Geometry check sheet. Reference: the model listing, model coordinates, mm. Face numbers are marked on the shaded views. A direction names the side the tool comes from. Round coordinates to 2 decimals unless told otherwise and drop trailing zeros. Write each loop counter-clockwise with the first axis right and the second up, starting at its lowest first coordinate (ties: lowest second). Pieces come first, ordered by that corner, then holes. Notation, with made-up numbers: M 74.25,-40 L 121.25,-40 A36 ccw 121.25,-3 Z; hole C 83.25,33 d11. An arc over 180 degrees is marked long. Use a Markdown table: item, result.
```python
from build123d import *

# Parameters (mm, degrees)
F0_W     = 25.4
F0_H     = 5.9481007091
F1_DEPTH = 12.7
F2_DEPTH = 25.4


with BuildPart() as f1:
    # F0 (on Front) → F1 (new body)
    with BuildSketch(Plane.XZ):
        with Locations((-12.7, 2.9740503545)):
            Rectangle(F0_W, F0_H)
        with BuildLine():
            Line((-25.4, 11.7354422192), (-25.4, 5.9481007091))
            Line((-25.4, 5.9481007091), (0, 5.9481007091))
            Line((0, 5.9481007091), (0, 11.7354422192))
            ThreePointArc((0, 11.7354422192), (-12.7, 24.4354422192), (-25.4, 11.7354422192))
        make_face()
    extrude(amount=-F1_DEPTH)

    # F0 (on Front) → F2 (join)
    with BuildSketch(Plane.XZ):
        with Locations((-12.7, 2.9740503545)):
            Rectangle(F0_W, F0_H)
    extrude(amount=F2_DEPTH)


solid = f1.part
```
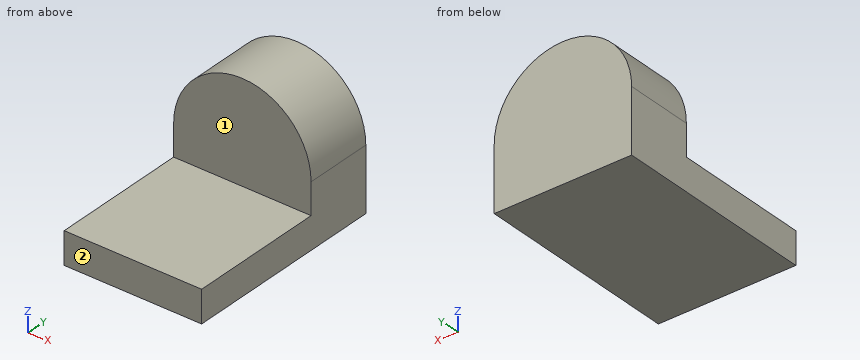
Item 1: Access from +Z, -Z, +X, -X, +Y, -Y to the whole of each face (thin tool, end or side, straight path). Record for the marked faces 1 and 2.
Outcome:
| item | result |
|---|---|
| face 1 | +Z, +X, -X, -Y |
| face 2 | +Z, -Z, +X, -X, -Y |
Item 2: Cross-section at C-C, the plane y = -7. Record the cut outline in (x, z).
Outcome:
| item | result |
|---|---|
| outline | M -25.4,0 L 0,0 L 0,5.95 L -25.4,5.95 Z |
Item 3: Material ranges on line 1 along Z through (x, y) = (-7.25, -7.5); line 2 along Y through (x, z) = (-1.25, 10); line 3 along Z through (x, y) = (-17.5, 3.5), recorded low to high. Write a range as from..to.
Outcome:
| item | result |
|---|---|
| line 1 | z = 0..5.95 |
| line 2 | y = 0..12.7 |
| line 3 | z = 0..23.49 |
Item 4: Cross-section at A-A, the plane x = -12.7. Record the cut outline in (y, z), and give its area (3 significant figures).
Outcome:
| item | result |
|---|---|
| outline | M -25.4,0 L 12.7,0 L 12.7,24.44 L 0,24.44 L 0,5.95 L -25.4,5.95 Z |
| area | 461 mm2 |
Item 5: Cross-section at D-D, the plane x = -4.5. Record the cut outline in (y, z).
Outcome:
| item | result |
|---|---|
| outline | M -25.4,0 L 12.7,0 L 12.7,21.43 L 0,21.43 L 0,5.95 L -25.4,5.95 Z |
Item 6: Cross-section at B-B, the plane z = 18. Record the cut outline in (x, y).
Outcome:
| item | result |
|---|---|
| outline | M -23.75,0 L -1.65,0 L -1.65,12.7 L -23.75,12.7 Z |
Item 7: Go/stop test with flat-tipped pins: pin 1 (1.5 mm diameter, centred on y = -11.5, z = 5.5, fed in from +X); pin 2 (4 mm diameter, centred on x = -15.5, z = 12.5, fed in from -Y). Record where each tip stops, or that it passes through.
Outcome:
| item | result |
|---|---|
| pin 1 | stops at x = 0 |
| pin 2 | stops at y = 0 |
